Design review of the part built by this model. Coordinates are the model's own, in mm. Face numbers are marked on the shaded views. Coordinates: 2 decimals unless noted, no trailing zeros. Loops run counter-clockwise (first coordinate to the right, second up) from the corner with the lowest first, then second, coordinate; pieces in that order, holes last. Notation, with made-up numbers: (48, -4.5) -> (71, -4.5) arc R31 cw to (71, 27.5) -> close; hole circle Ø1 at (-15.75, -14). An arc over 180 degrees is marked (long way). Answer as a JSON object with one key per item and string values.
```python
from build123d import *

# Parameters (mm, degrees)
THICKNESS_T = -5


with BuildPart() as part:
    # Sketch → Revolution (revolve)
    with BuildSketch(Plane.XZ):
        with BuildLine():
            Line((0, 0), (25, 0))
            Line((25, 0), (25, 52.470857))
            ThreePointArc((36.117714, 66.959745), (28.0997, 61.602279), (25, 52.470857))
            Line((36.117714, 66.959745), (40, 68))
            Line((40, 68), (40, 80))
            Line((40, 80), (0, 80))
            Line((0, 80), (0, 0))
        make_face()
    revolve(axis=Axis((0, 0, 0), (0, 0, 1)))

    # Thickness
    thickness_openings = [part.faces().sort_by_distance(p)[0] for p in [
        (0, 0, 80),
    ]]
    offset(amount=THICKNESS_T, openings=thickness_openings)


solid = part.part
```
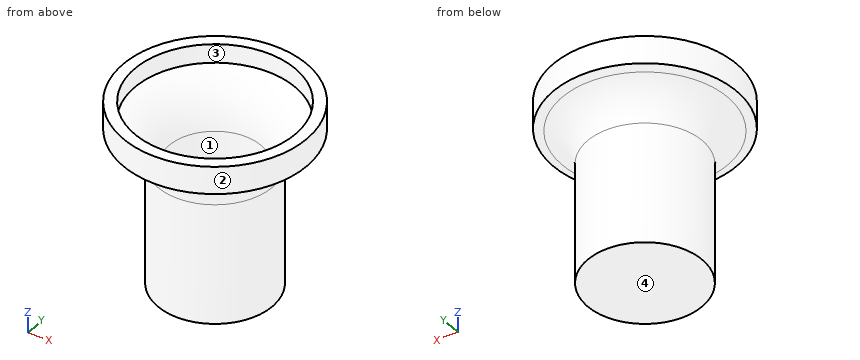
1) Wall thickness on probe 1 along Y at (x, z) = (0, 76); probe 2 along Y at (x, z) = (0, 34.5); probe 3 along Z at (x, y) = (-10, -2.5): over which ranges is each line inside the solid? List them lowest first.
Completed:
{"probe 1": "-40 to -35, 35 to 40", "probe 2": "-25 to -20, 20 to 25", "probe 3": "0 to 5"}
2) Add section C-C, the plane z = 42.5. Give the boundary of the cut face in (x, y), and give its area (3 significant figures).
Completed:
{"outline": "circle Ø50 at (0, 0); hole circle Ø40 at (0, 0)", "area": "707 mm²"}
3) The part is to be moulded in two halves that separate along Y. For the marked faces 1, 2, 3 and 4, say which applies: pulls with the +Y half, pulls with the -Y half, needs draft (parallel to the pull), parting line crosses it, or undercut.
Completed:
{"face 1": "undercut", "face 2": "parting line crosses it", "face 3": "undercut", "face 4": "needs draft"}
4) Add section A-A, the plane y = 0. Give the boundary of the cut face in (x, z).
Completed:
{"outline": "(-40, 68) -> (-36.12, 66.96) arc R15 cw to (-25, 52.47) -> (-25, 0) -> (25, 0) -> (25, 52.47) arc R15 cw to (36.12, 66.96) -> (40, 68) -> (40, 80) -> (35, 80) -> (35, 71.84) -> (34.82, 71.79) arc R20 ccw to (20, 52.47) -> (20, 5) -> (-20, 5) -> (-20, 52.47) arc R20 ccw to (-34.82, 71.79) -> (-35, 71.84) -> (-35, 80) -> (-40, 80) -> close"}
5) Clearance check with flat-ended pins moving along their axes: pin 1 Ø1 at (y, z) = (22, 21) entering from -X; pin 2 Ø20 at (x, y) = (1.5, -7.5) entering from +Z; pin 3 Ø4 at (y, z) = (16.5, 44) entering from -X. State where each tip first meets the part, or that it passes through.
Completed:
{"pin 1": "x = -12.76", "pin 2": "z = 5", "pin 3": "x = -20.37"}
6) Add section D-D, the plane z = 61.5. Give the boundary of the cut face in (x, y).
Completed:
{"outline": "circle Ø56.04 at (0, 0); hole circle Ø44.31 at (0, 0)"}
